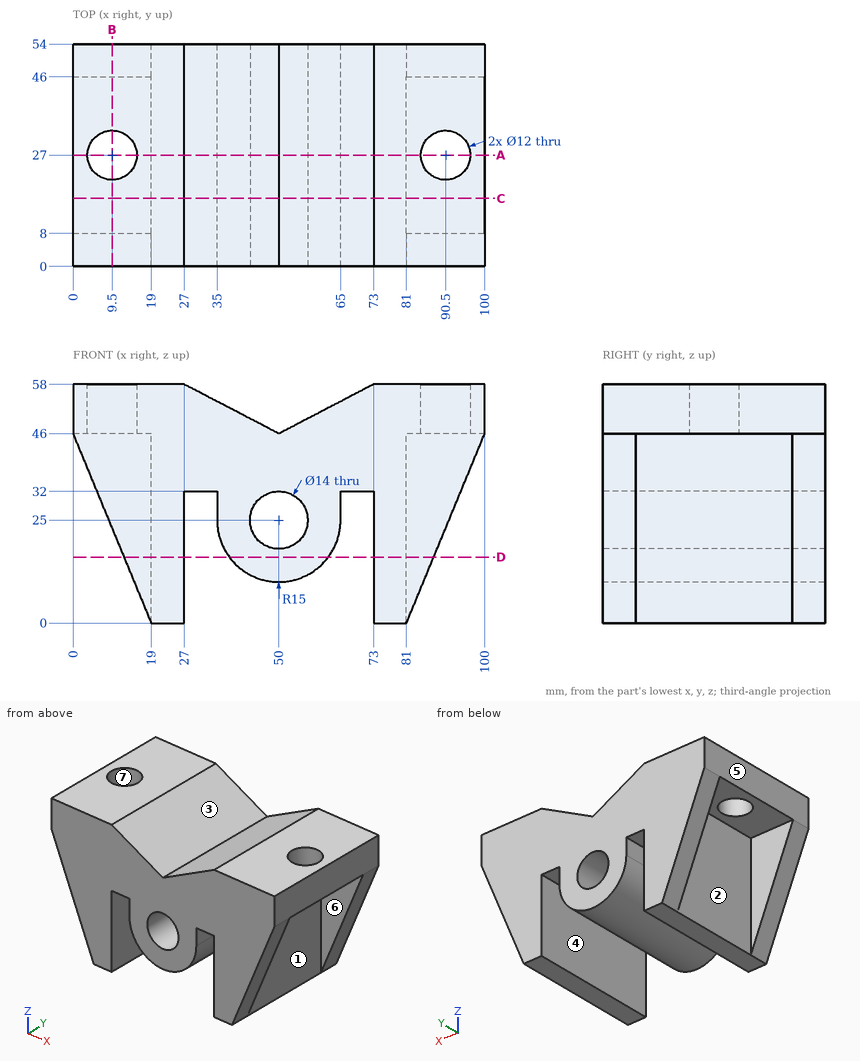
Design review of the part shown in the three views and the two pictorial views. Dimensions are in mm from the part's minimum x, y and z. A direction names the side the tool comes from. Give positions to 0.01 mm unless a question says otherwise; leave off trailing zeros. Loops run counter-clockwise (first coordinate to the right, second up) from the corner with the lowest first, then second, coordinate; pieces in that order, holes last. Notation, with made-up numbers: (83, 20.25) - (117, 20.25) arc R6 cw to (117, 30.25) - close; hole circle Ø9 at (-17, 2.25). An arc over 180 degrees is marked (long way). Answer as a JSON object with one key per item and string values.
Q1. Mouldability with a two-part tool opening along X and no side actions: class the marked faces 5, 6 and 7 as +X half, -X half, draft (parallel to the pull), parting line (faces both ways), or undercut.
Worked out:
{"face 5": "-X half", "face 6": "draft", "face 7": "undercut"}
Q2. To check wall thickness, follow line 1 along Y through (x, z) = (14.5, 29.5); line 2 along X through (y, z) = (29, 12); line 3 along Y through (x, z) = (9.5, 49.5). State the ranges of each line that lie inside material, in increasing order.
Worked out:
{"line 1": "y = 0 to 8, 46 to 54", "line 2": "x = 19 to 27, 42.52 to 57.48, 73 to 81", "line 3": "y = 0 to 21, 33 to 54"}
Q3. Add section B-B on x = 9.5. State the section outline as (y, z) points.
Worked out:
{"outline": "(0, 23) - (8, 23) - (8, 46) - (21, 46) - (21, 58) - (0, 58) - close; (33, 46) - (46, 46) - (46, 23) - (54, 23) - (54, 58) - (33, 58) - close"}
Q4. Insertion check: pin 1 (1.5 mm diameter, centred on x = 64.5, y = 21, fed in from -Z); pin 2 (5.5 mm diameter, centred on x = 10.5, z = 20, fed in from +Y); pin 3 (4 mm diameter, centred on x = 70.5, y = 25.5, fed in from -Z); pin 4 (12 mm diameter, centred on x = 54, y = 21.5, fed in from +Z). Each pin has a flat end and moves straight along its axis. Give the tip position at first contact, or say it passes through.
Worked out:
{"pin 1": "stops at z = 19.01", "pin 2": "stops at y = 54", "pin 3": "stops at z = 32", "pin 4": "stops at z = 51.22"}
Q5. For the marked faces 1, 2, 3 and 4, list the 3-axis set-ups (+Z, -Z, +X, -X, +Y, -Y) from which the entire face can be reached by the end or side of a thin tool; tool diameter is ignored.
Worked out:
{"face 1": "-Z, +X", "face 2": "-Z, -X", "face 3": "+Z, +Y, -Y", "face 4": "-Z, +Y, -Y"}
Q6. Add section C-C on y = 16.5. State the section outline as (x, z) points.
Worked out:
{"outline": "(0, 46) - (19, 46) - (19, 0) - (27, 0) - (27, 32) - (35, 32) - (35, 25) arc R15 ccw to (65, 25) - (65, 32) - (73, 32) - (73, 0) - (81, 0) - (81, 46) - (100, 46) - (100, 58) - (73, 58) - (50, 46) - (27, 58) - (0, 58) - close; hole circle Ø14 at (50, 25)"}
Q7. Add section D-D on z = 16. State the section outline as (x, y) points, plus the area to 3 significant figures.
Worked out:
{"outline": "(12.39, 0) - (27, 0) - (27, 54) - (12.39, 54) - (12.39, 46) - (19, 46) - (19, 8) - (12.39, 8) - close; (38, 0) - (62, 0) - (62, 54) - (38, 54) - close; (73, 0) - (87.61, 0) - (87.61, 8) - (81, 8) - (81, 46) - (87.61, 46) - (87.61, 54) - (73, 54) - close", "area": "2,370 mm^2"}
Q8. Add section A-A on y = 27. State the section outline as (x, z) points.
Worked out:
{"outline": "(0, 46) - (3.5, 46) - (3.5, 58) - (0, 58) - close; (15.5, 46) - (19, 46) - (19, 0) - (27, 0) - (27, 32) - (35, 32) - (35, 25) arc R15 ccw to (65, 25) - (65, 32) - (73, 32) - (73, 0) - (81, 0) - (81, 46) - (84.5, 46) - (84.5, 58) - (73, 58) - (50, 46) - (27, 58) - (15.5, 58) - close; (96.5, 46) - (100, 46) - (100, 58) - (96.5, 58) - close; hole circle Ø14 at (50, 25)"}
